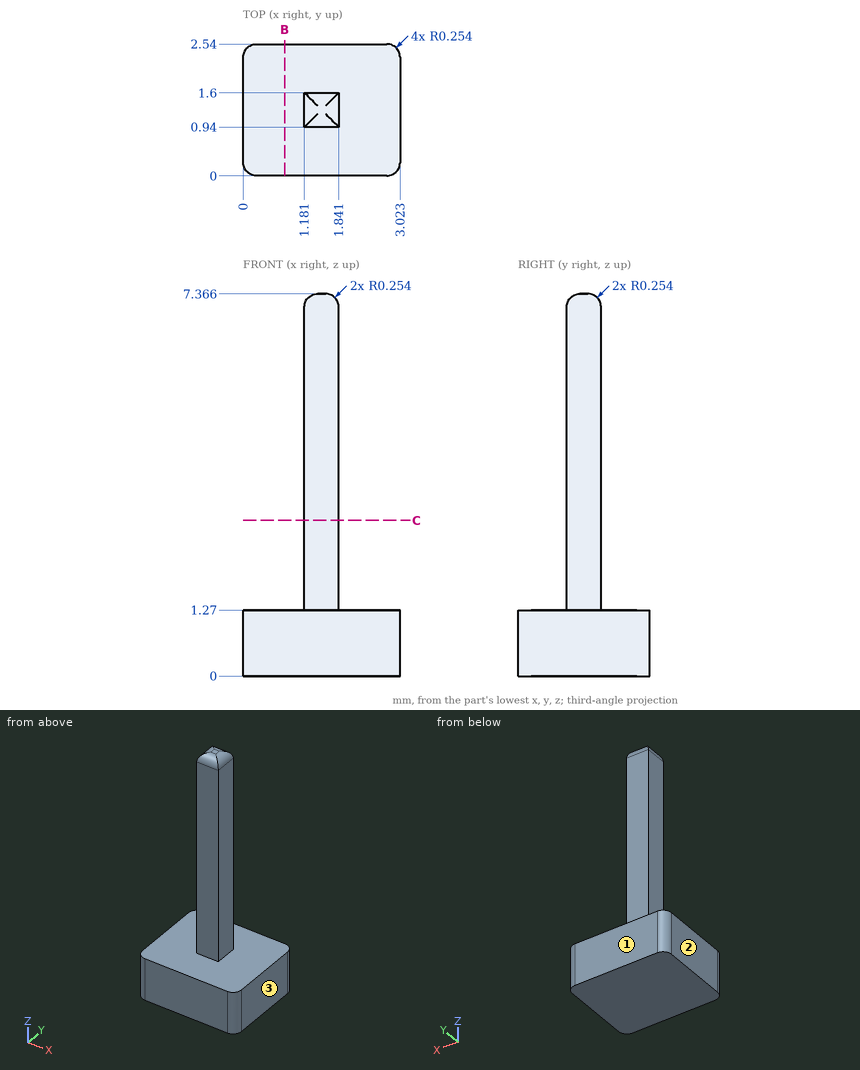
Can you work these out from the drawing? Everything is in mm from the part's minimum corner. Give positions to 0.01 mm unless a question says otherwise; leave off trailing zeros. Order: outer loops, then holes, each group sorted by start corner. A loop starts at its lowest first (then second) coordinate and runs counter-clockwise, first axis right, second up. Notation, with made-up numbers: M 41,-6 L 89,-6 A17 cw 89,14 Z; hole C 75,26 d8. An arc over 180 degrees is marked long. One line per item, written item: value.
Item 1: For pin 1 (0.5 mm diameter, centred on y = 1, z = 3.5, fed in from +X); pin 2 (0.5 mm diameter, centred on x = 1.5, z = 3, fed in from -Y), each with a flat end and sliding along its axis, tell me the tip position at first contact or that it passes through.
Verdict:
pin 1: x = 1.84
pin 2: y = 0.94
Item 2: Please list where these lines run through material, in increasing order: line 1 (Z direction, x = 2.65, y = 2); line 2 (Y direction, x = 1.5, z = 3.5); line 3 (X direction, y = 1.1, z = 6).
Verdict:
line 1: 0 to 1.27
line 2: 0.94 to 1.6
line 3: 1.18 to 1.84
Item 3: If we mould it in two halves opening along X, with no side actions, what happens to the marked faces 1, 2 and 3? For each: pulls with the +X half, pulls with the -X half, needs draft (parallel to the pull), parting line crosses it, or undercut.
Verdict:
face 1: needs draft
face 2: pulls with the -X half
face 3: pulls with the +X half
Item 4: If we section it at B-B on x = 0.8: Write out the boundary of the cut face in (y, z).
Verdict:
outline: M 0,0 L 2.54,0 L 2.54,1.27 L 0,1.27 Z
Item 5: If we section it at C-C on z = 3: Write out the boundary of the cut face in (x, y).
Verdict:
outline: M 1.18,0.94 L 1.84,0.94 L 1.84,1.6 L 1.18,1.6 Z
